Autodesk Inventor part; units mm, degrees
ref_plane "YZ Plane" through (0, 0, 0) normal (1, 0, 0) x (0, 1, 0)
ref_plane "XZ Plane" through (0, 0, 0) normal (0, 1, 0) x (-1, 0, 0)
ref_plane "XY Plane" through (0, 0, 0) normal (0, 0, 1) x (1, 0, 0)
sketch "Sketch1" plane through (0, 0, 0) normal (0, 0, 1) x (1, 0, 0)
  line L0 (-447.675, -1054.1) -> (447.675, -1054.1)
  line L1 (447.675, -1054.1) -> (447.675, 1054.1)
  line L2 (447.675, 1054.1) -> (-447.675, 1054.1)
  line L3 (-447.675, 1054.1) -> (-447.675, -1054.1)
  line L4 (-447.675, -1054.1) -> (447.675, 1054.1) construction
  line L5 (447.675, -1054.1) -> (-447.675, 1054.1) construction
  line L6 (-466.725, -1073.15) -> (466.725, -1073.15)
  line L7 (466.725, -1073.15) -> (466.725, 1073.15)
  line L8 (466.725, 1073.15) -> (-466.725, 1073.15)
  line L9 (-466.725, 1073.15) -> (-466.725, -1073.15)
  line L10 (-466.725, -1073.15) -> (466.725, 1073.15) construction
  line L11 (466.725, -1073.15) -> (-466.725, 1073.15) construction
  point P0 (0, 0)
  dimension "d0" = 895.35
  dimension "d1" = 2108.2
  dimension "d2" = 19.05
  dimension "d3" = 19.05
extrude "Extrusion1" add sketch "Sketch1" along normal blind 3.175
equation "\"d0\" = doorWidth"
equation "\"d1\" = doorHeight"
equation "\"wallThick\" = 44.45"
equation "\"roomWidth\" = 3048"
equation "\"roomDepth\" = 3657.6"
equation "\"roomHeight\" = 2438.4"
equation "\"doorWidth\" = 895.35"
equation "\"doorHeight\" = 2108.2"
equation "\"doorX\" = 774.7"
equation "\"doorY\" = 88.9"
equation "\"doorLip\" = 76.2"
equation "\"doorThick\" = 57.15"
equation "\"tubeD\" = 19.05"
equation "\"tubeTurnR\" = 76.2"
properties part number "door_rim"
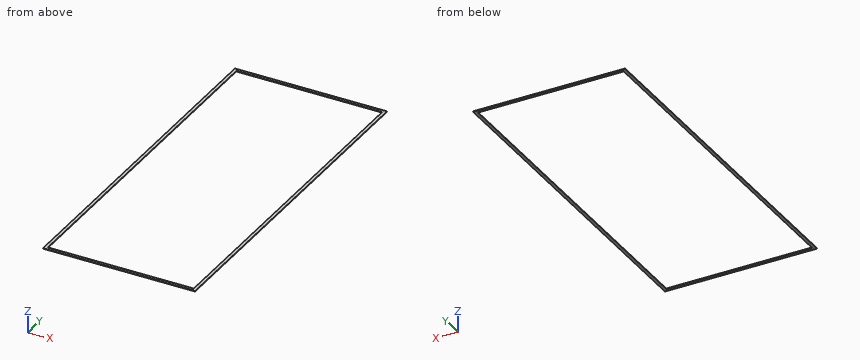
Input: part model. Units: mm. Frame: model coordinates. Round coordinates to 2 decimals unless told otherwise and drop trailing zeros. Order: outer loops, then holes, each group sorted by start corner. A loop starts at its lowest first (then second) coordinate and runs counter-clockwise, first axis right, second up. Notation, with made-up numbers: (24, 54.5) - (35, 54.5) arc R29 cw to (35, 76.5) - close; hole circle Ø3 at (38, 67). An arc over 180 degrees is marked (long way). Use a Markdown table: item, result.
1. Section A-A on z = 0.55. Return the cut outline in (x, y) (3 decimals), then the cut area to 3 significant figures.
Evaluation:
| item | result |
|---|---|
| outline | (-466.725, -1073.15) - (466.725, -1073.15) - (466.725, 1073.15) - (-466.725, 1073.15) - close; hole (-447.675, -1054.1) - (447.675, -1054.1) - (447.675, 1054.1) - (-447.675, 1054.1) - close |
| area | 116,000 mm^2 |
2. Section B-B on y = 150. Return the cut outline in (x, z) (3 decimals).
Evaluation:
| item | result |
|---|---|
| outline | (-466.725, 0) - (-447.675, 0) - (-447.675, 3.175) - (-466.725, 3.175) - close; (447.675, 0) - (466.725, 0) - (466.725, 3.175) - (447.675, 3.175) - close |
3. Section C-C on x = 95. Return the cut outline in (y, z) (3 decimals), then the cut area to 3 significant figures.
Evaluation:
| item | result |
|---|---|
| outline | (-1073.15, 0) - (-1054.1, 0) - (-1054.1, 3.175) - (-1073.15, 3.175) - close; (1054.1, 0) - (1073.15, 0) - (1073.15, 3.175) - (1054.1, 3.175) - close |
| area | 121 mm^2 |
4. Material intervals for probe 1 along Y at (x, z) = (291.5, 1.3); probe 2 along X at (y, z) = (-412, 1.25) (3 decimals), sorted ascending.
Evaluation:
| item | result |
|---|---|
| probe 1 | -1073.15 to -1054.1, 1054.1 to 1073.15 |
| probe 2 | -466.725 to -447.675, 447.675 to 466.725 |
